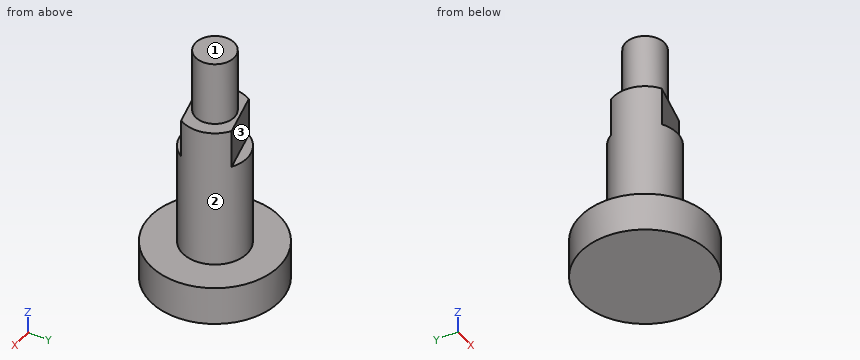
```python
from build123d import *

# Parameters (mm, degrees)
SKETCH1_R           = 5
BOSS_EXTRUDE1_DEPTH = 22
CUT_EXTRUDE1_START  = -6
CUT_EXTRUDE1_DEPTH  = 6
SKETCH3_R           = 3
BOSS_EXTRUDE2_DEPTH = 10
SKETCH4_R           = 10
BOSS_EXTRUDE3_DEPTH = 6


with BuildPart() as part:
    # Sketch1 → Boss-Extrude1 (new body)
    with BuildSketch(Plane.XY):
        Circle(SKETCH1_R)
    extrude(amount=BOSS_EXTRUDE1_DEPTH)

    # Sketch2 → Cut-Extrude1 (cut)
    with BuildSketch(Plane.XY.offset(22).offset(CUT_EXTRUDE1_START)):
        with BuildLine():
            Line((2.638277831, 4.247292089), (-4.299208102, 2.552804281))
            ThreePointArc((-4.299208102, 2.552804281), (-1.186378765, 4.857211693), (2.638277831, 4.247292089))
        make_face()
        with BuildLine():
            Line((-2.638277831, -4.247292089), (4.299208102, -2.552804281))
            ThreePointArc((4.299208102, -2.552804281), (1.186378765, -4.857211693), (-2.638277831, -4.247292089))
        make_face()
    extrude(amount=CUT_EXTRUDE1_DEPTH, mode=Mode.SUBTRACT)

    # Sketch3 → Boss-Extrude2 (add)
    with BuildSketch(Plane.XY.offset(22)):
        Circle(SKETCH3_R)
    extrude(amount=BOSS_EXTRUDE2_DEPTH)

    # Sketch4 → Boss-Extrude3 (add)
    with BuildSketch(Plane(origin=(0, 0, 0), x_dir=(-1, 0, 0), z_dir=(0, 0, -1))):
        Circle(SKETCH4_R)
    extrude(amount=BOSS_EXTRUDE3_DEPTH)


solid = part.part
```
Source: CAD feature listing. Evaluate the final solid. Frame: model axes, mm. Face numbers are marked on the shaded views. A direction names the side the tool comes from. Give positions to 0.01 mm unless a question says otherwise; leave off trailing zeros. Write each loop counter-clockwise with the first axis right and the second up, starting at its lowest first coordinate (ties: lowest second). Pieces come first, ordered by that corner, then holes. Notation, with made-up numbers: (43, 72) - (93, 72) arc R25 ccw to (93, 93) - close; hole circle Ø3 at (56, 55). An arc over 180 degrees is marked (long way). One line per item, written item: value. Start each with the question number.
Q1. Section query D-D, the plane x = -2. Return the cut outline in (y, z), then the cut area to 3 significant figures.
Q2. First-contact query: pin 1 Ø10 at (y, z) = (-4, 15) entering from -X; pin 2 Ø6 at (y, z) = (-7, 16.5) entering from -X; pin 3 Ø1.5 at (x, z) = (-4, 13.5) entering from +Y. Flat tips, straight axial feed; report the tip coordinate or a pass-through.
Q3. Section query C-C, the plane z = 24. Return the cut outline in (x, y), then the cut area to 3 significant figures.
Q4. Section query A-A, the plane y = 0. Return the cut outline in (x, z).
Q5. Section query B-B, the plane x = 0. Return the cut outline in (y, z).
Q6. Material intervals for probe 1 along Z at (x, y) = (-3, 1.75); probe 2 along Y at (x, z) = (0, 22.5); probe 3 along Z at (x, y) = (2, -7.25), sorted ascending. Write a range as from..to.
Q7. Set-up query: the marked faces 1, 2 and 3. Return all of +Z, -Z, +X, -X, +Y, -Y with unobstructed straight access to the full face (end or side cutting, diameter ignored); none if empty.
Answer:
1. outline: (-9.8, -6) - (9.8, -6) - (9.8, 0) - (4.58, 0) - (4.58, 16) - (3.11, 16) - (3.11, 22) - (2.24, 22) - (2.24, 32) - (-2.24, 32) - (-2.24, 22) - (-4.09, 22) - (-4.09, 16) - (-4.58, 16) - (-4.58, 0) - (-9.8, 0) - close
1. area: 352 mm2
2. pin 1: stops at x = -5
2. pin 2: stops at x = -3
2. pin 3: stops at y = 3.8
3. outline: circle Ø6 at (0, 0)
3. area: 28.3 mm2
4. outline: (-10, -6) - (10, -6) - (10, 0) - (5, 0) - (5, 22) - (3, 22) - (3, 32) - (-3, 32) - (-3, 22) - (-5, 22) - (-5, 0) - (-10, 0) - close
5. outline: (-10, -6) - (10, -6) - (10, 0) - (5, 0) - (5, 16) - (3.6, 16) - (3.6, 22) - (3, 22) - (3, 32) - (-3, 32) - (-3, 22) - (-3.6, 22) - (-3.6, 16) - (-5, 16) - (-5, 0) - (-10, 0) - close
6. probe 1: z = -6..22
6. probe 2: y = -3..3
6. probe 3: z = -6..0
7. face 1: +Z, +X, -X, +Y, -Y
7. face 2: +Z
7. face 3: +Z, -X, +Y
